Autodesk Inventor part; units mm, degrees
ref_plane "YZ Plane" through (0, 0, 0) normal (1, 0, 0) x (0, 1, 0)
ref_plane "XZ Plane" through (0, 0, 0) normal (0, 1, 0) x (-1, 0, 0)
ref_plane "XY Plane" through (0, 0, 0) normal (0, 0, 1) x (1, 0, 0)
sketch "スケッチ1" plane through (0, 0, 0) normal (0, 0, 1) x (1, 0, 0)
  circle A0 centre (104.0735, 2) radius 6.025
  arc A1 (100.4168, -2.7885) -> (70.6822, 5.0468) centre (76.1402, -34.5791) ccw
  line L0 (69.7806, -5) -> (104.0735, 2) construction
  circle A2 centre (69.7806, -5) radius 5 construction
  arc A3 (102.7574, -3.8795) -> (72.4739, -9.2126) centre (94.0202, -42.9136) ccw construction
  circle A4 centre (75.3506, 22) radius 5 construction
  circle A5 centre (70, 10) radius 1.5
  circle A6 centre (70, 10) radius 5
  arc A7 (109.4834, 4.652) -> (75.6055, 26.9935) centre (73.5667, -12.9545) ccw construction
  arc A8 (108.1244, 6.4599) -> (68.3957, 14.7356) centre (81.2303, -23.1494) ccw
  arc A9 (105.8851, 7.7462) -> (66.341, -1.371) centre (93.8576, -30.4027) ccw construction
  line L1 (70, 10) -> (104.0735, 2) construction
  circle A10 centre (82.0403, 11.2819) radius 1.5
  line L2 (48.483, 55.1333) -> (82.5564, 47.1333) construction
  line L3 (82.5564, 47.1333) -> (53.8336, 67.1333) construction
  line L4 (82.5564, 47.1333) -> (48.2636, 40.1333) construction
  circle A11 centre (53.8336, 67.1333) radius 5 construction
  circle A12 centre (48.2636, 40.1333) radius 5 construction
  circle A13 centre (48.483, 55.1333) radius 5
  circle A14 centre (82.5564, 47.1333) radius 1.5
  circle A15 centre (82.5564, 47.1333) radius 5
  circle A16 centre (48.483, 55.1333) radius 1.5
  arc A17 (77.6092, 46.4087) -> (54.8703, 62.242) centre (58.8098, 43.6549) ccw construction
  arc A18 (78.225, 44.6356) -> (51.2502, 50.9689) centre (61.7656, 35.1441) ccw
  arc A19 (79.6686, 43.0516) -> (52.5201, 37.51) centre (68.6948, 27.5411) ccw construction
  arc A20 (85.2716, 51.3319) -> (44.1201, 42.9319) centre (68.9807, 26.1405) ccw construction
  arc A21 (86.7799, 49.8095) -> (45.8918, 59.4095) centre (61.4389, 33.7524) ccw
  arc A22 (87.4691, 48.0636) -> (53.0017, 72.0636) centre (57.993, 42.4818) ccw construction
  circle A23 centre (82.5564, 47.1333) radius 4
  circle A24 centre (104.0735, 2) radius 4
  circle A25 centre (70, 10) radius 4
  point P0 (0, 0)
  point P1 (0, 0)
  point P2 (0, 0)
  dimension "d0" = 40
  dimension "d1" = 10
  dimension "d2" = 40
  dimension "d3" = 10
  dimension "d4" = 10
  dimension "d5" = 3
  dimension "d6" = 19
  dimension "d7" = 30
  dimension "d8" = 3
  dimension "d9" = 8
  dimension "d10" = 8
  dimension "d11" = 8
extrude "押し出し1" add sketch "スケッチ1" along normal blind 3 contours A0 | A0 A1 A6 A8 | A6
properties part number "heikousita" material "アルミニウム 2014-T4"
CAD build for the part. Positions are in the model's coordinates, mm. Give positions to 0.01 mm unless a question says otherwise; leave off trailing zeros. Loops run counter-clockwise (first coordinate to the right, second up) from the corner with the lowest first, then second, coordinate; pieces in that order, holes last. Notation, with made-up numbers: (51, 31) -> (82, 31) arc R12 cw to (82, 36) -> close; hole circle Ø11 at (83.25, 63). An arc over 180 degrees is marked (long way). Use a Markdown table: item, result.
1. Mould opens along X. For faces 1 (the cylindrical face through (107.89, 0.8, 1.48)), 2 (the cylindrical face through (108.78, -1.76, 1.48)), 3 (the flat face through (87, 9, 0)) say: pulls with the +X half, pulls with the -X half, needs draft (parallel to the pull), parting line crosses it, or undercut.
Check result:
| item | result |
|---|---|
| face 1 | undercut |
| face 2 | parting line crosses it |
| face 3 | needs draft |
2. Wall check: L1, parallel to X at y = 1, z = 2.35; L2, parallel to X at y = 9.75, z = 0.5; L3, parallel to Y at x = 70, z = 2.4. Give the ranges that are in metal, low to high. Write a range as [from, to].
Check result:
| item | result |
|---|---|
| L1 | x = [94.42, 100.2], [107.95, 110.01] |
| L2 | x = [65.01, 66.01], [73.99, 103.98] |
| L3 | y = [5, 6], [14, 15.24] |
3. Flat gauge pins, fed straight in: pin 1 (1.5 mm diameter, centred on y = 12.5, z = 1, fed in from +X); pin 2 (1 mm diameter, centred on y = 13.5, z = 1, fed in from +X). Where does each tip first touch, or does it go through?
Check result:
| item | result |
|---|---|
| pin 1 | stops at x = 100.78 |
| pin 2 | stops at x = 98.35 |
4. Slice it at B-B (y = 2). List the corners of the cut face in (x, z), plus the area to 3 significant figures.
Check result:
| item | result |
|---|---|
| outline | (92.33, 0) -> (100.07, 0) -> (100.07, 3) -> (92.33, 3) -> close; (108.07, 0) -> (110.1, 0) -> (110.1, 3) -> (108.07, 3) -> close |
| area | 29.3 mm^2 |
5. Slice it at D-D (x = 98.5). List the corners of the cut face in (y, z), plus the area to 3 significant figures.
Check result:
| item | result |
|---|---|
| outline | (-1.41, 0) -> (12.93, 0) -> (12.93, 3) -> (-1.41, 3) -> close |
| area | 43.0 mm^2 |
6. Slice it at C-C (z = 0.9). Give the number of separate pieces and of enclosed holes in the cut face, plus the area to 3 significant figures.
Check result:
| item | result |
|---|---|
| separate pieces | 1 |
| enclosed holes | 3 |
| area | 420 mm^2 |
7. Slice it at A-A (x = 106). List the corners of the cut face in (y, z), plus the area to 3 significant figures.
Check result:
| item | result |
|---|---|
| outline | (-3.71, 0) -> (-1.51, 0) -> (-1.51, 3) -> (-3.71, 3) -> close; (5.51, 0) -> (8.26, 0) -> (8.26, 3) -> (5.51, 3) -> close |
| area | 14.9 mm^2 |
